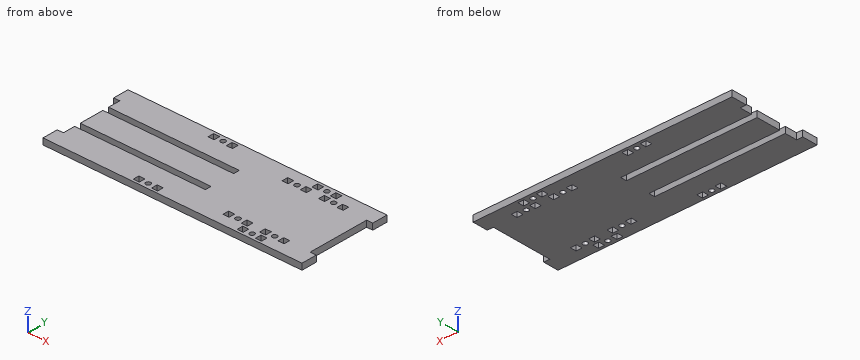
from build123d import *

# Parameters (mm, degrees)
ESQUISSE1_W        = 5
ESQUISSE1_H        = 5
ESQUISSE1_R        = 2
BOSS_EXTRU_1_DEPTH = 5


with BuildPart() as part:
    # Esquisse1 → Boss.-Extru.1 (new body)
    with BuildSketch(Plane.XY):
        Polygon((162, 37.65), (0, 37.65), (-50, 37.65), (-50, 25), (-45, 25), (-45, 15), (62, 15), (62, 10), (0, 10), (-45, 10), (-45, -10), (62, -10), (62, -15), (-45, -15), (-45, -25), (-50, -25), (-50, -37.65), (0, -37.65), (162, -37.65), (162, -25), (157, -25), (157, 25), (162, 25), align=None)
        with Locations((24.5, -33.15)):
            Rectangle(ESQUISSE1_W, ESQUISSE1_H, mode=Mode.SUBTRACT)
        with Locations((32, -33.15)):
            Circle(ESQUISSE1_R, mode=Mode.SUBTRACT)
        with Locations((39.5, -33.15)):
            Rectangle(ESQUISSE1_W, ESQUISSE1_H, mode=Mode.SUBTRACT)
        with Locations((91.5, -26.15)):
            Rectangle(ESQUISSE1_W, ESQUISSE1_H, mode=Mode.SUBTRACT)
        with Locations((99, -26.15)):
            Circle(ESQUISSE1_R, mode=Mode.SUBTRACT)
        with Locations((106.5, -26.15)):
            Rectangle(ESQUISSE1_W, ESQUISSE1_H, mode=Mode.SUBTRACT)
        with Locations((109.5, -33.15)):
            Rectangle(ESQUISSE1_W, ESQUISSE1_H, mode=Mode.SUBTRACT)
        with Locations((117, -33.15)):
            Circle(ESQUISSE1_R, mode=Mode.SUBTRACT)
        with Locations((124.5, -33.15)):
            Rectangle(ESQUISSE1_W, ESQUISSE1_H, mode=Mode.SUBTRACT)
        with Locations((121.5, -26.15)):
            Rectangle(ESQUISSE1_W, ESQUISSE1_H, mode=Mode.SUBTRACT)
        with Locations((129, -26.15)):
            Circle(ESQUISSE1_R, mode=Mode.SUBTRACT)
        with Locations((136.5, -26.15)):
            Rectangle(ESQUISSE1_W, ESQUISSE1_H, mode=Mode.SUBTRACT)
        with Locations((24.5, 33.15)):
            Rectangle(ESQUISSE1_W, ESQUISSE1_H, mode=Mode.SUBTRACT)
        with Locations((32, 33.15)):
            Circle(ESQUISSE1_R, mode=Mode.SUBTRACT)
        with Locations((39.5, 33.15)):
            Rectangle(ESQUISSE1_W, ESQUISSE1_H, mode=Mode.SUBTRACT)
        with Locations((91.5, 26.15)):
            Rectangle(ESQUISSE1_W, ESQUISSE1_H, mode=Mode.SUBTRACT)
        with Locations((99, 26.15)):
            Circle(ESQUISSE1_R, mode=Mode.SUBTRACT)
        with Locations((106.5, 26.15)):
            Rectangle(ESQUISSE1_W, ESQUISSE1_H, mode=Mode.SUBTRACT)
        with Locations((121.5, 26.15)):
            Rectangle(ESQUISSE1_W, ESQUISSE1_H, mode=Mode.SUBTRACT)
        with Locations((129, 26.15)):
            Circle(ESQUISSE1_R, mode=Mode.SUBTRACT)
        with Locations((136.5, 26.15)):
            Rectangle(ESQUISSE1_W, ESQUISSE1_H, mode=Mode.SUBTRACT)
        with Locations((109.5, 33.15)):
            Rectangle(ESQUISSE1_W, ESQUISSE1_H, mode=Mode.SUBTRACT)
        with Locations((117, 33.15)):
            Circle(ESQUISSE1_R, mode=Mode.SUBTRACT)
        with Locations((124.5, 33.15)):
            Rectangle(ESQUISSE1_W, ESQUISSE1_H, mode=Mode.SUBTRACT)
    extrude(amount=BOSS_EXTRU_1_DEPTH)


solid = part.part
Geometry: final body of the model. Coordinates: model frame, mm. Round coordinates to 2 decimals unless told otherwise and drop trailing zeros. Order: outer loops, then holes, each group sorted by start corner. A loop starts at its lowest first (then second) coordinate and runs counter-clockwise, first axis right, second up. Notation, with made-up numbers: (34, -3.75) -> (77, -3.75) arc R16 ccw to (77, 27.25) -> close; hole circle Ø9 at (55.5, 25). An arc over 180 degrees is marked (long way). Put each result on its own line as item: value. Start each with the question number.
Q1. Section D-D on x = 92. Return the cut outline in (y, z), and give its area (4 significant figures).
Q2. Section A-A on x = 117. Return the cut outline in (y, z), and give its area (4 significant figures).
Q3. First-contact query: pin 1 (1 mm diameter, centred on y = 8.5, z = 3, fed in from -X). Flat tip, straight axial feed; report the tip coordinate or a pass-through.
Q4. Section C-C on x = 32. Return the cut outline in (y, z).
Q5. Section B-B on y = -33.15. Return the cut outline in (x, z), and give its area (3 significant figures).
Q6. Line query: probe 1 along Y at (x, z) = (19.5, 4.65); probe 2 along Y at (x, z) = (99, 2.15); probe 3 along Y at (x, z) = (32, 1.35). Output: solid intervals per line, ascending.
Ans:
1. outline: (-37.65, 0) -> (-28.65, 0) -> (-28.65, 5) -> (-37.65, 5) -> close; (-23.65, 0) -> (23.65, 0) -> (23.65, 5) -> (-23.65, 5) -> close; (28.65, 0) -> (37.65, 0) -> (37.65, 5) -> (28.65, 5) -> close
1. area: 326.5 mm2
2. outline: (-37.65, 0) -> (-35.15, 0) -> (-35.15, 5) -> (-37.65, 5) -> close; (-31.15, 0) -> (31.15, 0) -> (31.15, 5) -> (-31.15, 5) -> close; (35.15, 0) -> (37.65, 0) -> (37.65, 5) -> (35.15, 5) -> close
2. area: 336.5 mm2
3. pin 1: stops at x = -45
4. outline: (-37.65, 0) -> (-35.15, 0) -> (-35.15, 5) -> (-37.65, 5) -> close; (-31.15, 0) -> (-15, 0) -> (-15, 5) -> (-31.15, 5) -> close; (-10, 0) -> (10, 0) -> (10, 5) -> (-10, 5) -> close; (15, 0) -> (31.15, 0) -> (31.15, 5) -> (15, 5) -> close; (35.15, 0) -> (37.65, 0) -> (37.65, 5) -> (35.15, 5) -> close
5. outline: (-50, 0) -> (22, 0) -> (22, 5) -> (-50, 5) -> close; (27, 0) -> (30, 0) -> (30, 5) -> (27, 5) -> close; (34, 0) -> (37, 0) -> (37, 5) -> (34, 5) -> close; (42, 0) -> (107, 0) -> (107, 5) -> (42, 5) -> close; (112, 0) -> (115, 0) -> (115, 5) -> (112, 5) -> close; (119, 0) -> (122, 0) -> (122, 5) -> (119, 5) -> close; (127, 0) -> (162, 0) -> (162, 5) -> (127, 5) -> close
5. area: 920 mm2
6. probe 1: y = -37.65 to -15, -10 to 10, 15 to 37.65
6. probe 2: y = -37.65 to -28.15, -24.15 to 24.15, 28.15 to 37.65
6. probe 3: y = -37.65 to -35.15, -31.15 to -15, -10 to 10, 15 to 31.15, 35.15 to 37.65
